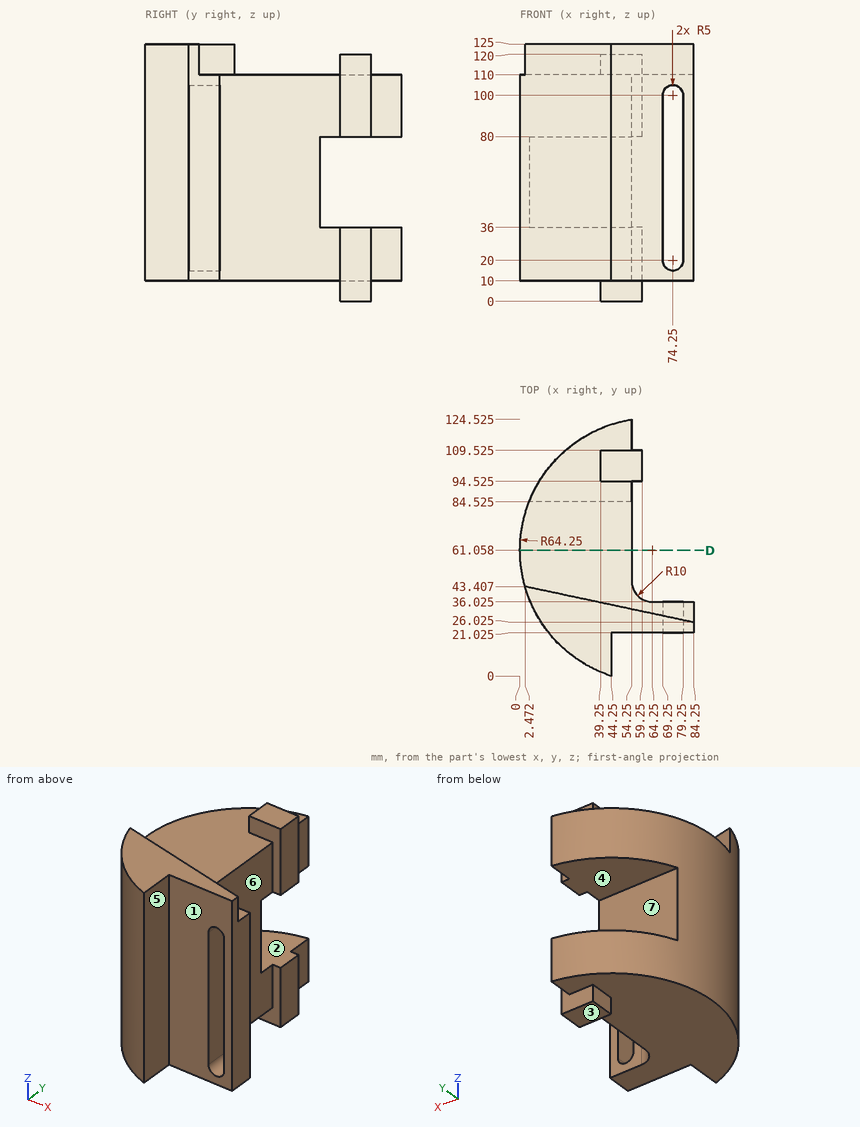
Answer from the drawing. Dimensions are ordinates in mm from the lowest x, y and z of the part. A direction names the side the tool comes from. Give positions to 0.01 mm unless a question says otherwise; leave off trailing zeros. Order: outer loops, then holes, each group sorted by start corner. A loop starts at its lowest first (then second) coordinate and runs counter-clockwise, first axis right, second up. Notation, with made-up numbers: (86, 1) -> (144, 1) arc R32 cw to (144, 37) -> close; hole circle Ø10 at (8, 11). An arc over 180 degrees is marked (long way). Answer as a JSON object with one key per item and string values. Group by question number.
1. A tool of negligible diameter and unlimited length cuts with its end or side. For the marked faces 5, 6 and 7, from which of +Z, -Z, +X, -X, +Y, -Y can it reach the whole face along a straight path? Write none if from no direction.
2. Section D-D on y = 61 is taken. Determine the outline of the cut face in (x, z).
3. The mould has two halves that part along Z. Classify the marked faces 1, 2, 3 and 4: released by +Z, released by -Z, zero draft, split by the parting line, or undercut.
4. Flat-ended cylindrical pins translate along their axes: pin 1 Ø1.5 at (x, z) = (26, 101.5) entering from -Y; pin 2 Ø4.5 at (y, z) = (115, 90.5) entering from +X; pin 3 Ø12 at (x, z) = (20.5, 72) entering from -Y. Find the tip coordinate at first contact, or state that the pin passes through.
5. Consider line 1 along Z through (x, y) = (12, 98); line 2 along Z through (x, y) = (44, 18); line 3 along Z through (x, y) = (15.5, 47.5). Determine where each line is inside the solid, lowest interval first. Write a range as [from, to].
Result sheet:
{
 "1": {"face 5": "+Z, -Z, +X, -Y", "face 6": "+Z, -Z, +X", "face 7": "+X, -X, +Y"},
 "2": {"outline": "(0, 10) -> (54.25, 10) -> (54.25, 110) -> (0, 110) -> close"},
 "3": {"face 1": "zero draft", "face 2": "undercut", "face 3": "released by -Z", "face 4": "undercut"},
 "4": {"pin 1": "stops at y = 8.89", "pin 2": "stops at x = 54.25", "pin 3": "stops at y = 9.07"},
 "5": {"line 1": "z = [10, 36], [80, 110]", "line 2": "z = [10, 125]", "line 3": "z = [10, 110]"}
}
